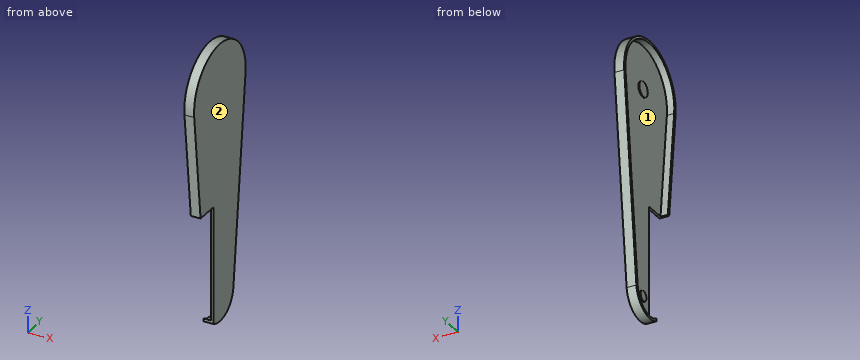
```python
from build123d import *

# Parameters (mm, degrees)
DODANIE_WYCI_GNI_CIE1_DEPTH = 5
DODANIE_WYCI_GNI_CIE2_START = 15
DODANIE_WYCI_GNI_CIE2_DEPTH = 15
SZKIC3_R                    = 10.56077606
SZKIC3_R_2                  = 15.572635527
DODANIE_WYCI_GNI_CIE3_DEPTH = 2
WYTNIJ_WYCI_GNI_CIE1_START  = -20
WYTNIJ_WYCI_GNI_CIE1_DEPTH  = 20


# Read off the part's stored shape, not the designer's step: Wytnij-wyci_gni_cie1
with BuildPart() as part:
    # Szkic1 → Dodanie-wyci_gni_cie1 (new body)
    with BuildSketch(Plane(origin=(0, 0, 0), x_dir=(0, 0, -1), z_dir=(1, 0, 0))):
        with BuildLine():
            Line((10.058823529, 94.465973076), (430.294117647, 49.718933198))
            ThreePointArc((430.294117647, 49.718933198), (475, 0), (430.294117647, -49.718933198))
            Line((430.294117647, -49.718933198), (10.058823529, -94.465973076))
            ThreePointArc((10.058823529, -94.465973076), (-95, 0), (10.058823529, 94.465973076))
        make_face()
    extrude(amount=DODANIE_WYCI_GNI_CIE1_DEPTH)

    # Szkic2 → Dodanie-wyci_gni_cie2 (add)
    with BuildSketch(Plane.ZY.offset(DODANIE_WYCI_GNI_CIE2_START)):
        with BuildLine():
            Line((-10.058823529, 94.465973076), (-430.294117647, 49.718933198))
            ThreePointArc((-430.294117647, 49.718933198), (-475, 0), (-430.294117647, -49.718933198))
            Line((-430.294117647, -49.718933198), (-10.058823529, -94.465973076))
            ThreePointArc((-10.058823529, -94.465973076), (95, 0), (-10.058823529, 94.465973076))
        make_face()
        with BuildLine():
            Line((-9.529411765, 89.494079756), (-429.764705882, 44.747039878))
            ThreePointArc((-429.764705882, 44.747039878), (-470, 0), (-429.764705882, -44.747039878))
            Line((-429.764705882, -44.747039878), (-9.529411765, -89.494079756))
            ThreePointArc((-9.529411765, -89.494079756), (90, 0), (-9.529411765, 89.494079756))
        make_face(mode=Mode.SUBTRACT)
    extrude(amount=-DODANIE_WYCI_GNI_CIE2_DEPTH)

    # Szkic3 → Dodanie-wyci_gni_cie3 (add)
    with BuildSketch(Plane.ZY):
        with Locations(Location((-425, 0, 0), (0, 0, 180))):
            Circle(SZKIC3_R)
        with Locations(Location((0, 0, 0), (0, 0, 180))):
            Circle(SZKIC3_R_2)
    extrude(amount=DODANIE_WYCI_GNI_CIE3_DEPTH)

    # Wytnij-wyci_gni_cie1 outline → Wytnij-wyci_gni_cie1 (cut)
    with BuildSketch(Plane(origin=(5, 0, 0), x_dir=(0, 0, -1), z_dir=(1, 0, 0)).offset(WYTNIJ_WYCI_GNI_CIE1_START)):
        with BuildLine():
            ThreePointArc((430.294117647, -49.718933198), (452.973624228, -41.442446206), (469.131245302, -23.503897297))
            Line((469.131245302, -23.503897297), (229.084460246, -23.503897297))
            Line((229.084460246, -23.503897297), (229.084460246, -71.143922221))
            Line((229.084460246, -71.143922221), (430.294117647, -49.718933198))
        make_face()
    extrude(amount=WYTNIJ_WYCI_GNI_CIE1_DEPTH, mode=Mode.SUBTRACT)


solid = part.part
```
Geometry check sheet. Reference: the model listing, model coordinates, mm. Face numbers are marked on the shaded views. Give positions to 0.01 mm unless a question says otherwise; leave off trailing zeros. Order: outer loops, then holes, each group sorted by start corner. A loop starts at its lowest first (then second) coordinate and runs counter-clockwise, first axis right, second up.
1. Thickness scan on L1, parallel to Y at x = -10.75, z = 0; L2, parallel to Z at x = -9.75, y = 0; L3, parallel to X at y = 11.5, z = 72. Record the ranges inside material, lowest first.
2. Section check B-B, the plane z = 0. Enter the section's corners in (x, y), and give its area (3 significant figures).
3. Gauge pin test, flat ends, axial feed: pin 1 Ø10 at (x, z) = (1, -134) entering from -Y; pin 2 Ø10 at (x, z) = (-8.5, -313) entering from -Y; pin 3 Ø10 at (x, z) = (-12, -40.5) entering from +Y. Record the tip position at first contact, or that the pin passes through.
4. Section check A-A, the plane y = 0. Enter the section's corners in (x, z).
5. Section check D-D, the plane y = -76. Enter the section's corners in (x, z), and give its area (3 significant figures).
6. Release check for a two-part mould opening along Z. For the marked faces 1 and 2 record: pulls with the +Z half, pulls with the -Z half, needs draft (parallel to the pull), parting line crosses it, or undercut.
7. Section check C-C, the plane x = -8.75. Enter the section's corners in (y, z).
Values follow:
1. L1: y = -95 to -90, 90 to 95
1. L2: z = -475 to -470, 90 to 95
1. L3: x = 0 to 5
2. outline: (-15, -95) - (5, -95) - (5, 95) - (-15, 95) - (-15, 90) - (0, 90) - (0, 15.57) - (-2, 15.57) - (-2, -15.57) - (0, -15.57) - (0, -90) - (-15, -90) - close
2. area: 1,160 mm2
3. pin 1: stops at y = -81.8
3. pin 2: stops at y = 56.65
3. pin 3: stops at y = 91.76
4. outline: (-15, -475) - (5, -475) - (5, 95) - (-15, 95) - (-15, 90) - (0, 90) - (0, 15.57) - (-2, 15.57) - (-2, -15.57) - (0, -15.57) - (0, -414.44) - (-2, -414.44) - (-2, -435.56) - (0, -435.56) - (0, -470) - (-15, -470) - close
5. outline: (-15, -183.48) - (5, -183.48) - (5, 57) - (-15, 57) - (-15, 48.21) - (0, 48.21) - (0, -136.26) - (-15, -136.26) - close
5. area: 2,040 mm2
6. face 1: undercut
6. face 2: needs draft
7. outline: (-94.47, -10.06) - (-71.14, -229.08) - (-66.12, -229.08) - (-89.49, -9.53) arc R90 cw (long way) to (89.49, -9.53) - (44.75, -429.76) arc R45 cw to (-23.5, -463.37) - (-23.5, -469.13) arc R50 ccw to (49.72, -430.29) - (94.47, -10.06) arc R95 ccw (long way) to start
